Input: part model. Units: mm. Frame: model coordinates. Face numbers are marked on the shaded views. A direction names the side the tool comes from. Give positions to 0.01 mm unless a question says otherwise; leave off trailing zeros. Write each loop counter-clockwise with the first axis right and the second up, starting at its lowest first coordinate (ties: lowest second). Pieces come first, ordered by that corner, then holes. Notation, with made-up numbers: (64, 79) - (86, 79) arc R21 cw to (86, 99) - close; hole circle Ø9 at (89.5, -27). An arc over 180 degrees is marked (long way). Use a Markdown table: item, result. Add a question column.
1. Material intervals for probe 1 along X at (y, z) = (2.05, -11.5) (3 decimals); probe 2 along X at (y, z) = (3.65, -5) (3 decimals); probe 3 along Z at (x, y) = (46, 3), sorted ascending.
2. Pin query (flat end, axial travel): pin 1 (10 mm diameter, centred on y = -26, z = -4.5, fed in from -X); pin 2 (3.5 mm diameter, centred on x = 46.5, z = -35, fed in from -Y); pin 3 (10 mm diameter, centred on y = -48.5, z = -22.5, fed in from +X); pin 4 (1.6 mm diameter, centred on x = 1, y = -51.5, fed in from -Z). Return the tip coordinate at first contact, or that it passes through.
3. Section query A-A, the plane z = -28.5. Return loops of the section in (x, y) (3 decimals), plus the area to 3 significant figures.
4. Section query D-D, the plane x = 12.5. Return loops of the section in (y, z) (3 decimals), plus the area to 3 significant figures.
5. Section query B-B, the plane x = 39. Return loops of the section in (y, z).
6. Set-up query: the marked faces 1 and 2. Return all of +Z, -Z, +X, -X, +Y, -Y with unobstructed straight access to the full face (end or side cutting, diameter ignored); none if empty.
7. Section query C-C, the plane z = -9. Return loops of the section in (x, y), plus the area to 3 significant figures.
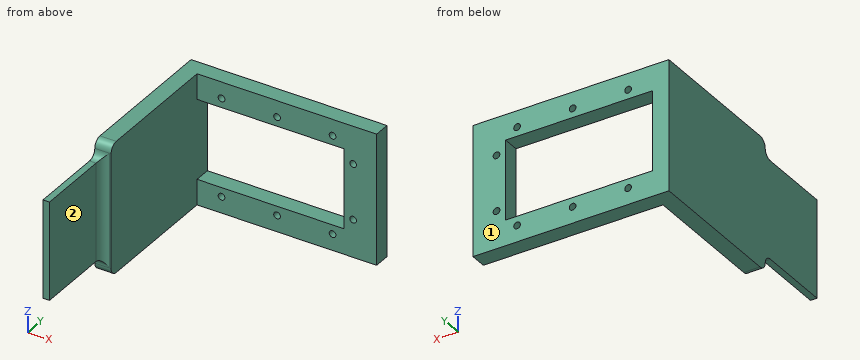
```python
from build123d import *

# Parameters (mm, degrees)
SKETCH1_W           = 60
SKETCH1_H           = 40
SKETCH1_W_2         = 45
SKETCH1_H_2         = 24.4
BOSS_EXTRUDE1_DEPTH = 5
SKETCH6_W           = 5
SKETCH6_H           = 40
BOSS_EXTRUDE4_DEPTH = 41.5
SKETCH7_W           = 2
SKETCH7_H           = 30
BOSS_EXTRUDE5_DEPTH = 25
FILLET2_R           = 2.5
FILLET3_R           = 2.5
CUT_EXTRUDE1_REACH  = 100.093
SKETCH8_R           = 1.025


with BuildPart() as part:
    # Sketch1 → Boss-Extrude1 (new body)
    with BuildSketch(Plane(origin=(0, 0, 0), x_dir=(1, 0, 0), z_dir=(0, 1, 0))):
        with Locations((30, 20)):
            Rectangle(SKETCH1_W, SKETCH1_H)
        with Locations((27.5, 20)):
            Rectangle(SKETCH1_W_2, SKETCH1_H_2, mode=Mode.SUBTRACT)
    extrude(amount=BOSS_EXTRUDE1_DEPTH)

    # Sketch6 → Boss-Extrude4 (add)
    with BuildSketch(Plane.XZ):
        with Locations((2.5, -20)):
            Rectangle(SKETCH6_W, SKETCH6_H)
    extrude(amount=BOSS_EXTRUDE4_DEPTH)

    # Sketch7 → Boss-Extrude5 (add)
    with BuildSketch(Plane(origin=(0, -41.5, 0), x_dir=(-1, 0, 0), z_dir=(0, -1, 0))):
        with Locations((-1, 20)):
            Rectangle(SKETCH7_W, SKETCH7_H)
    extrude(amount=BOSS_EXTRUDE5_DEPTH)

    # Fillet2
    fillet2_edges = [part.edges().sort_by_distance(p)[0] for p in [
        (2, -41.5, -20),
    ]]
    fillet(fillet2_edges, radius=FILLET2_R)

    # Fillet3
    fillet3_edges = [part.edges().sort_by_distance(p)[0] for p in [
        (2.25, -41.5, -5),
        (2.25, -41.5, -35),
        (2.5, -41.5, 0),
        (2.5, -41.5, -40),
    ]]
    fillet(fillet3_edges, radius=FILLET3_R - 0.0001)  # a hair under: the kernel refuses the full size

    # Sketch8 → Cut-Extrude1 (cut, up to next)
    with BuildSketch(Plane(origin=(0, 0, 0), x_dir=(-1, 0, 0), z_dir=(0, -1, 0)), mode=Mode.PRIVATE) as cut_extrude1_sk1:
        with Locations(Location((-46.5, 5, 0), (0, 0, 90))):
            Circle(SKETCH8_R)
    cut_extrude1_tool1 = extrude(cut_extrude1_sk1.sketch, amount=-CUT_EXTRUDE1_REACH, mode=Mode.PRIVATE) & part.part
    # Sketch8 → Cut-Extrude1 (cut, up to next)
    with BuildSketch(Plane(origin=(0, 0, 0), x_dir=(-1, 0, 0), z_dir=(0, -1, 0)), mode=Mode.PRIVATE) as cut_extrude1_sk2:
        with Locations(Location((-29.5, 5, 0), (0, 0, 90))):
            Circle(SKETCH8_R)
    cut_extrude1_tool2 = extrude(cut_extrude1_sk2.sketch, amount=-CUT_EXTRUDE1_REACH, mode=Mode.PRIVATE) & part.part
    # Sketch8 → Cut-Extrude1 (cut, up to next)
    with BuildSketch(Plane(origin=(0, 0, 0), x_dir=(-1, 0, 0), z_dir=(0, -1, 0)), mode=Mode.PRIVATE) as cut_extrude1_sk3:
        with Locations(Location((-12.5, 5, 0), (0, 0, 90))):
            Circle(SKETCH8_R)
    cut_extrude1_tool3 = extrude(cut_extrude1_sk3.sketch, amount=-CUT_EXTRUDE1_REACH, mode=Mode.PRIVATE) & part.part
    # Sketch8 → Cut-Extrude1 (cut, up to next)
    with BuildSketch(Plane(origin=(0, 0, 0), x_dir=(-1, 0, 0), z_dir=(0, -1, 0)), mode=Mode.PRIVATE) as cut_extrude1_sk4:
        with Locations(Location((-52.8, 11.5, 0), (0, 0, 90))):
            Circle(SKETCH8_R)
    cut_extrude1_tool4 = extrude(cut_extrude1_sk4.sketch, amount=-CUT_EXTRUDE1_REACH, mode=Mode.PRIVATE) & part.part
    # Sketch8 → Cut-Extrude1 (cut, up to next)
    with BuildSketch(Plane(origin=(0, 0, 0), x_dir=(-1, 0, 0), z_dir=(0, -1, 0)), mode=Mode.PRIVATE) as cut_extrude1_sk5:
        with Locations(Location((-12.5, 35, 0), (0, 0, 90))):
            Circle(SKETCH8_R)
    cut_extrude1_tool5 = extrude(cut_extrude1_sk5.sketch, amount=-CUT_EXTRUDE1_REACH, mode=Mode.PRIVATE) & part.part
    # Sketch8 → Cut-Extrude1 (cut, up to next)
    with BuildSketch(Plane(origin=(0, 0, 0), x_dir=(-1, 0, 0), z_dir=(0, -1, 0)), mode=Mode.PRIVATE) as cut_extrude1_sk6:
        with Locations(Location((-29.5, 35, 0), (0, 0, 90))):
            Circle(SKETCH8_R)
    cut_extrude1_tool6 = extrude(cut_extrude1_sk6.sketch, amount=-CUT_EXTRUDE1_REACH, mode=Mode.PRIVATE) & part.part
    # Sketch8 → Cut-Extrude1 (cut, up to next)
    with BuildSketch(Plane(origin=(0, 0, 0), x_dir=(-1, 0, 0), z_dir=(0, -1, 0)), mode=Mode.PRIVATE) as cut_extrude1_sk7:
        with Locations(Location((-46.5, 35, 0), (0, 0, 90))):
            Circle(SKETCH8_R)
    cut_extrude1_tool7 = extrude(cut_extrude1_sk7.sketch, amount=-CUT_EXTRUDE1_REACH, mode=Mode.PRIVATE) & part.part
    # Sketch8 → Cut-Extrude1 (cut, up to next)
    with BuildSketch(Plane(origin=(0, 0, 0), x_dir=(-1, 0, 0), z_dir=(0, -1, 0)), mode=Mode.PRIVATE) as cut_extrude1_sk8:
        with Locations(Location((-52.8, 28.5, 0), (0, 0, 90))):
            Circle(SKETCH8_R)
    cut_extrude1_tool8 = extrude(cut_extrude1_sk8.sketch, amount=-CUT_EXTRUDE1_REACH, mode=Mode.PRIVATE) & part.part
    add(cut_extrude1_tool1.solids().sort_by_distance((46.5, 0, -5))[0], mode=Mode.SUBTRACT)
    add(cut_extrude1_tool2.solids().sort_by_distance((29.5, 0, -5))[0], mode=Mode.SUBTRACT)
    add(cut_extrude1_tool3.solids().sort_by_distance((12.5, 0, -5))[0], mode=Mode.SUBTRACT)
    add(cut_extrude1_tool4.solids().sort_by_distance((52.8, 0, -11.5))[0], mode=Mode.SUBTRACT)
    add(cut_extrude1_tool5.solids().sort_by_distance((12.5, 0, -35))[0], mode=Mode.SUBTRACT)
    add(cut_extrude1_tool6.solids().sort_by_distance((29.5, 0, -35))[0], mode=Mode.SUBTRACT)
    add(cut_extrude1_tool7.solids().sort_by_distance((46.5, 0, -35))[0], mode=Mode.SUBTRACT)
    add(cut_extrude1_tool8.solids().sort_by_distance((52.8, 0, -28.5))[0], mode=Mode.SUBTRACT)


solid = part.part
```
Result sheet:
| question | item | result |
|---|---|---|
| 1 | probe 1 | x = 0 to 5, 50 to 51.775, 53.825 to 60 |
| 1 | probe 2 | x = 0 to 11.475, 13.525 to 28.475, 30.525 to 45.475, 47.525 to 60 |
| 1 | probe 3 | z = -40 to -35.89, -34.11 to -32.2, -7.8 to -5.89, -4.11 to 0 |
| 2 | pin 1 | stops at x = 0 |
| 2 | pin 2 | stops at y = 0 |
| 2 | pin 3 | stops at x = 2.05 |
| 2 | pin 4 | stops at z = -35 |
| 3 | outline | (0, -66.5) - (2, -66.5) - (2, -44) arc R2.5 cw to (4.5, -41.5) - (5, -41.5) - (5, 5) - (0, 5) - close; (50, 0) - (51.775, 0) - (51.775, 5) - (50, 5) - close; (53.825, 0) - (60, 0) - (60, 5) - (53.825, 5) - close |
| 3 | area | 324 mm² |
| 4 | outline | (0, -40) - (5, -40) - (5, -36.025) - (0, -36.025) - close; (0, -33.975) - (5, -33.975) - (5, -32.2) - (0, -32.2) - close; (0, -7.8) - (5, -7.8) - (5, -6.025) - (0, -6.025) - close; (0, -3.975) - (5, -3.975) - (5, 0) - (0, 0) - close |
| 4 | area | 57.5 mm² |
| 5 | outline | (0, -40) - (5, -40) - (5, -32.2) - (0, -32.2) - close; (0, -7.8) - (5, -7.8) - (5, 0) - (0, 0) - close |
| 6 | face 1 | +Z, -Z, +X, -X, +Y |
| 6 | face 2 | +Z, -Z, +X, -Y |
| 7 | outline | (0, -66.5) - (2, -66.5) - (2, -44) arc R2.5 cw to (4.5, -41.5) - (5, -41.5) - (5, 5) - (0, 5) - close; (50, 0) - (60, 0) - (60, 5) - (50, 5) - close |
| 7 | area | 334 mm² |
